```python
from build123d import *

# Parameters (mm, degrees)
F1_DEPTH        = 22.225
F3_D            = 23.415625
F4_D            = 26.67
F4_DEPTH        = 12.7
F4_TIP          = 8.0124763547
F5_W            = 19.05
F5_H            = 22.225
F6_DEPTH        = 3.175
F8_D            = 11.1125
F8_DEPTH        = 25.4
F8_TIP          = 3.3385318145
F9_D            = 13.716
F9_DEPTH        = 9.525
F9_TIP          = 4.1207021253
F11_D           = 9
F11_CBORE_D     = 14.5
F11_CBORE_DEPTH = 10


with BuildPart() as f1:
    # F0 (on Front) → F1 (new body)
    with BuildSketch(Plane.XZ):
        Polygon((-9.525, 20.6375), (-36.5125, 9.525), (-36.5125, -9.525), (-9.525, -20.6375), (9.525, -20.6375), (36.5125, -9.525), (36.5125, 9.525), (9.525, 20.6375), align=None)
    extrude(amount=-F1_DEPTH)

    # F3 (through all)
    with Locations(Plane.XZ):
        with Locations((0, 0)):
            Hole(F3_D / 2)

    # F4
    with Locations(Plane.XZ):
        with Locations((0, 0)):
            Hole(F4_D / 2, depth=F4_DEPTH)
            with Locations((0, 0, -(F4_DEPTH + F4_TIP / 2))):  # 118° drill point
                Cone(0, F4_D / 2, F4_TIP, mode=Mode.SUBTRACT)

    # F5 (on face) → F6 (join)
    with BuildSketch(Plane.XY.offset(20.6375)):
        with Locations((0, 11.1125)):
            Rectangle(F5_W, F5_H)
    extrude(amount=F6_DEPTH)

    # F8
    with Locations(Plane.XY.offset(23.8125)):
        with Locations((0, 12.7)):
            Hole(F8_D / 2, depth=F8_DEPTH)
            with Locations((0, 0, -(F8_DEPTH + F8_TIP / 2))):  # 118° drill point
                Cone(0, F8_D / 2, F8_TIP, mode=Mode.SUBTRACT)

    # F9
    with Locations(Plane.XY.offset(23.8125)):
        with Locations((0, 12.7)):
            Hole(F9_D / 2, depth=F9_DEPTH)
            with Locations((0, 0, -(F9_DEPTH + F9_TIP / 2))):  # 118° drill point
                Cone(0, F9_D / 2, F9_TIP, mode=Mode.SUBTRACT)

    # F11 (through all)
    with Locations(Plane.XZ):
        with Locations((-25, 0), (25, 0)):
            CounterBoreHole(F11_D / 2, F11_CBORE_D / 2, F11_CBORE_DEPTH)


solid = f1.part
```
Here's how the part is built. I have some questions about the finished solid (model axes, mm). A direction names the side the tool comes from. Give positions to 0.01 mm unless a question says otherwise; leave off trailing zeros. Order: outer loops, then holes, each group sorted by start corner. A loop starts at its lowest first (then second) coordinate and runs counter-clockwise, first axis right, second up. Notation, with made-up numbers: (59, 24) -> (86, 24) arc R26 cw to (86, 47) -> close; hole circle Ø2 at (32, -12). An arc over 180 degrees is marked (long way). Use CSV: the item, a comma, the result in double quotes. Start each with the question number.
Item 1: Thinking about a two-plate mould opening in X: for faces 1 (the flat face through (-23.208, 10.957, -15.003)), 2 (the cylindrical face through (2.54, 18.01, -11.43)), 3 (the flat face through (8, 22.225, 11)), which applies, pulls with the +X half, pulls with the -X half, needs draft (parallel to the pull), parting line crosses it, or undercut?
Item 2: Suppose I cut it at D-D (z = 19). List the corners of the cut face in (x, y) for me (3 decimals).
Item 3: If I drill on probe 1 along X at (y, z) = (21, -4); probe 2 along Z at (x, y) = (6, 12.25); probe 3 along Y at (x, z) = (-1, 15.5) (3 decimals), over which ranges is the centre line in solid material (lowest first)? Write a range as [from, to].
Item 4: On a 3-axis mill with a long thin cutter (end or side, diameter ignored), from which of +Z, -Z, +X, -X, +Y, -Y can I reach the whole of each face in a straight line? I mean faces 4 (the flat face through (9.525, 11, 22)), 5 (the cylindrical face through (2.89, 6.44, -13.02)), 6 (the flat face through (-9.525, 11, 22)). Say none if no direction works.
Item 5: Suppose I cut it at A-A (z = 0). Give the number of separate pieces and of enclosed holes in the cut face, and give its area (3 significant figures).
Item 6: Suppose I cut it at C-C (x = 21.5). List the corners of the cut face in (y, z) for me (3 decimals).
Item 7: I'm going to push flat-ended pins straight in: P1, Ø2, axis at x = 2.5, y = 12, coming from the +Z side; P2, Ø1, axis at y = 11.5, z = 23, coming from the +X side (3 decimals); P3, Ø7, axis at x = 23.5, z = -0.5, coming from the -Y side. Where does each tip first touch, or does it pass through?
Answer block:
1,face 1,"pulls with the -X half"
1,face 2,"undercut"
1,face 3,"needs draft"
2,outline,"(-13.502, 0) -> (13.502, 0) -> (13.502, 22.225) -> (-13.502, 22.225) -> close; hole circle Ø13.716 at (0, 12.7)"
3,probe 1,"x = [-36.51, -27.06], [-22.94, -11], [11, 22.94], [27.06, 36.51]"
3,probe 2,"z = [-20.64, -11.91], [11.91, 13.78]"
3,probe 3,"y = [0, 5.915], [19.485, 22.225]"
4,face 4,"+Z, +X, +Y, -Y"
4,face 5,"-Y"
4,face 6,"+Z, -X, +Y, -Y"
5,separate pieces,"4"
5,enclosed holes,"0"
5,area,"550 mm^2"
6,outline,"(0, -15.707) -> (22.225, -15.707) -> (22.225, -2.828) -> (10, -2.828) -> (10, -6.349) -> (0, -6.349) -> close; (0, 6.349) -> (10, 6.349) -> (10, 2.828) -> (22.225, 2.828) -> (22.225, 15.707) -> (0, 15.707) -> close"
7,P1,"stops at z = -12.58"
7,P2,"stops at x = 9.525"
7,P3,"stops at y = 10"
